For this review, take the finished solid that the model builds, in its own axes (mm). A direction names the side the tool comes from. Give positions to 0.01 mm unless a question says otherwise; leave off trailing zeros. Loops run counter-clockwise (first coordinate to the right, second up) from the corner with the lowest first, then second, coordinate; pieces in that order, holes last.
```python
from build123d import *

# Parameters (mm, degrees)
F0_W     = 185
F0_H     = 94
F0_W_2   = 193
F0_H_2   = 10
F0_H_3   = 5
F1_DEPTH = 4.5
F2_DEPTH = 5


# Not quite as in the source:
# - a feature names something its author has since deleted; it is built from what else it names


with BuildPart() as f1:
    # F0 (on Top) → F1 (new body)
    with BuildSketch(Plane.XY):
        Polygon((96.5, 52), (96.5, 56), (-96.5, 56), (-96.5, 52), (-96.5, -42), (-96.5, -46), (96.5, -46), (96.5, -42), align=None)
        with Locations((0, 5)):
            Rectangle(F0_W, F0_H, mode=Mode.SUBTRACT)
        with Locations((0, 5)):
            Rectangle(F0_W, F0_H)
        with Locations((0, -51)):
            Rectangle(F0_W_2, F0_H_2)
        with Locations((0, 58.5)):
            Rectangle(F0_W_2, F0_H_3)
    extrude(amount=-F1_DEPTH)

    # F0 (on Top) → F2 (join)
    with BuildSketch(Plane.XY):
        Polygon((96.5, 52), (96.5, 56), (-96.5, 56), (-96.5, 52), (-96.5, -42), (-96.5, -46), (96.5, -46), (96.5, -42), align=None)
        with Locations((0, 5)):
            Rectangle(F0_W, F0_H, mode=Mode.SUBTRACT)
    extrude(amount=F2_DEPTH)


solid = f1.part
```
Q1. For probe 1 along Y at (x, z) = (38, 3); probe 2 along X at (y, z) = (37, 2.75); probe 3 along Z at (x, y) = (14, -18), list the stretches that pass through material, from the lowest coordinate up.
Answers:
probe 1: y = -46 to -42, 52 to 56
probe 2: x = -96.5 to -92.5, 92.5 to 96.5
probe 3: z = -4.5 to 0
Q2. Consider section B-B on y = -4. Give the boundary of the cut face in (x, z), plus the area to 4 significant figures.
Answers:
outline: (-96.5, -4.5) - (96.5, -4.5) - (96.5, 5) - (92.5, 5) - (92.5, 0) - (-92.5, 0) - (-92.5, 5) - (-96.5, 5) - close
area: 908.5 mm2
Q3. For pin 1 Ø6 at (x, y) = (-49.5, -30.5) entering from +Z; pin 2 Ø2.5 at (x, z) = (9, 3) entering from -Y; pin 3 Ø5.5 at (x, z) = (25, 1.5) entering from +Y; pin 4 Ø2.5 at (x, z) = (-10, 3.5) entering from +Y, all flat-tipped, find the tip position at first contact; note any pin that passes through.
Answers:
pin 1: stops at z = 0
pin 2: stops at y = -46
pin 3: stops at y = 61
pin 4: stops at y = 56
Q4. Consider section A-A on x = -4. Give the boundary of the cut face in (y, z), plus the area to 4 significant figures.
Answers:
outline: (-56, -4.5) - (61, -4.5) - (61, 0) - (56, 0) - (56, 5) - (52, 5) - (52, 0) - (-42, 0) - (-42, 5) - (-46, 5) - (-46, 0) - (-56, 0) - close
area: 566.5 mm2
Q5. Machinability: for faces 4 (the flat face through (-1, 59, 0)), 5 (the flat face through (-92.5, 4, 2)), 6 (the flat face through (-1, 61, -2)), 7 (the flat face through (-1, -46, 2)), which of the approach directions +Z, -Z, +X, -X, +Y, -Y give a long, thin tool a straight path to every point of the face, cutting with its end or side? Answer none if there is none.
Answers:
face 4: +Z, +X, -X, +Y
face 5: +Z
face 6: +Z, -Z, +X, -X, +Y
face 7: +Z, +X, -X, -Y
Q6. Mouldability with a two-part tool opening along Y and no side actions: class faces 1 (the flat face through (-1, 6, 0)), 2 (the flat face through (-1, -51, 0)), 3 (the flat face through (1, 56, 2)) as +Y half, -Y half, draft (parallel to the pull), parting line (faces both ways), or undercut.
Answers:
face 1: undercut
face 2: draft
face 3: +Y half
